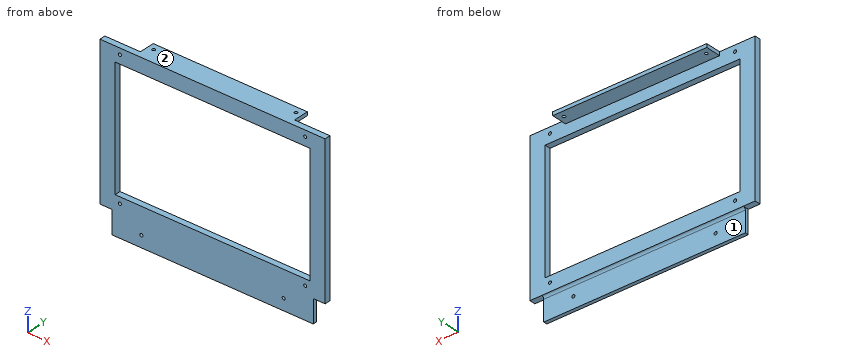
from build123d import *

# Parameters (mm, degrees)
SKETCH1_W           = 170
SKETCH1_H           = 146
BOSS_EXTRUDE1_DEPTH = 3
SKETCH2_R           = 1.3
CUT_EXTRUDE1_DEPTH  = 3
CUT_EXTRUDE2_DEPTH  = 3
BOSS_EXTRUDE2_START = 2
SKETCH4_R           = 1.3
SKETCH4_W           = 164.3
SKETCH4_H           = 101.7
BOSS_EXTRUDE2_DEPTH = 2
BOSS_EXTRUDE5_DEPTH = 10
SKETCH10_W          = 126.5
SKETCH10_H          = 5
BOSS_EXTRUDE6_DEPTH = 10
SKETCH12_W          = 190
SKETCH12_H          = 3
BOSS_EXTRUDE8_DEPTH = 13
SKETCH13_R          = 1.3
CUT_EXTRUDE3_DEPTH  = 13
FILLET4_R           = 2
SKETCH14_R          = 1.3
CUT_EXTRUDE4_DEPTH  = 13
SKETCH15_W          = 30
SKETCH15_H          = 3
CUT_EXTRUDE5_DEPTH  = 13


with BuildPart() as part:
    # Sketch1 → Boss-Extrude1 (new body)
    with BuildSketch(Plane(origin=(0, 0, 0), x_dir=(1, 0, 0), z_dir=(0, 1, 0))):
        Rectangle(SKETCH1_W, SKETCH1_H)
    extrude(amount=BOSS_EXTRUDE1_DEPTH)

    # Sketch2 → Cut-Extrude1 (cut)
    with BuildSketch(Plane(origin=(0, 3, 0), x_dir=(1, 0, 0), z_dir=(0, 1, 0))):
        with Locations(Location((78.15, -67.9, 0), (0, 0, 270))):
            Circle(SKETCH2_R)
        with Locations(Location((-78.15, 46.4, 0), (0, 0, 270))):
            Circle(SKETCH2_R)
        with Locations(Location((-78.15, -67.9, 0), (0, 0, 270))):
            Circle(SKETCH2_R)
        with Locations(Location((78.15, 46.4, 0), (0, 0, 270))):
            Circle(SKETCH2_R)
    extrude(amount=-CUT_EXTRUDE1_DEPTH, mode=Mode.SUBTRACT)

    # Sketch3 → Cut-Extrude2 (cut)
    with BuildSketch(Plane(origin=(0, 3, 0), x_dir=(1, 0, 0), z_dir=(0, 1, 0))):
        Polygon((-78.15, -60.6), (-82.15, -60.6), (-82.15, 41.1), (-78.15, 41.1), (78.15, 41.1), (82.15, 41.1), (82.15, -60.6), (78.15, -60.6), align=None)
    extrude(amount=-CUT_EXTRUDE2_DEPTH, mode=Mode.SUBTRACT)

    # Sketch4 → Boss-Extrude2 (add)
    with BuildSketch(Plane(origin=(0, 3, 0), x_dir=(1, 0, 0), z_dir=(0, 1, 0)).offset(BOSS_EXTRUDE2_START)):
        Polygon((-82.15, 53.5), (85, 53.5), (85, -73), (-85, -73), (-85, 53.5), align=None)
        with Locations(Location((-78.15, 46.4, 0), (0, 0, 270))):
            Circle(SKETCH4_R, mode=Mode.SUBTRACT)
        with Locations(Location((-78.15, -67.9, 0), (0, 0, 270))):
            Circle(SKETCH4_R, mode=Mode.SUBTRACT)
        with Locations(Location((78.15, -67.9, 0), (0, 0, 270))):
            Circle(SKETCH4_R, mode=Mode.SUBTRACT)
        with Locations(Location((78.15, 46.4, 0), (0, 0, 270))):
            Circle(SKETCH4_R, mode=Mode.SUBTRACT)
        with Locations((0, -9.75)):
            Rectangle(SKETCH4_W, SKETCH4_H, mode=Mode.SUBTRACT)
    extrude(amount=-BOSS_EXTRUDE2_DEPTH)

    # Sketch9 → Boss-Extrude5 (add)
    with BuildSketch(Plane.ZY.offset(85)):
        Polygon((-53.5, 3), (-53.5, 5), (73, 5), (73, 0), (-53.5, 0), align=None)
    extrude(amount=BOSS_EXTRUDE5_DEPTH)

    # Sketch10 → Boss-Extrude6 (add)
    with BuildSketch(Plane(origin=(85, 0, 0), x_dir=(0, 0, -1), z_dir=(1, 0, 0))):
        with Locations((-9.75, 2.5)):
            Rectangle(SKETCH10_W, SKETCH10_H)
    extrude(amount=BOSS_EXTRUDE6_DEPTH)

    # Sketch12 → Boss-Extrude8 (add)
    with BuildSketch(Plane(origin=(0, 5, 0), x_dir=(1, 0, 0), z_dir=(0, 1, 0))):
        with Locations((0, -71.5)):
            Rectangle(SKETCH12_W, SKETCH12_H)
    extrude(amount=BOSS_EXTRUDE8_DEPTH)

    # Sketch13 → Cut-Extrude3 (cut)
    with BuildSketch(Plane(origin=(0, 3, 0), x_dir=(1, 0, 0), z_dir=(0, 1, 0))):
        with Locations(Location((-60, 63.25, 0), (0, 0, 270))):
            Circle(SKETCH13_R)
        with Locations(Location((60, 63.25, 0), (0, 0, 270))):
            Circle(SKETCH13_R)
    extrude(amount=-CUT_EXTRUDE3_DEPTH, mode=Mode.SUBTRACT)

    # Fillet4
    fillet4_edges = [part.edges().sort_by_distance(p)[0] for p in [
        (0, 3, -53.5),
    ]]
    fillet(fillet4_edges, radius=FILLET4_R - 0.0001)  # a hair under: the kernel refuses the full size

    # Sketch14 → Cut-Extrude4 (cut)
    with BuildSketch(Plane(origin=(0, 0, 70), x_dir=(-1, 0, 0), z_dir=(0, 0, -1))):
        with Locations((-60, 12.5)):
            Circle(SKETCH14_R)
        with Locations((60, 12.5)):
            Circle(SKETCH14_R)
    extrude(amount=-CUT_EXTRUDE4_DEPTH, mode=Mode.SUBTRACT)

    # Sketch15 → Cut-Extrude5 (cut)
    with BuildSketch(Plane(origin=(0, 18, 0), x_dir=(1, 0, 0), z_dir=(0, 1, 0))):
        with Locations((80, -71.5)):
            Rectangle(SKETCH15_W, SKETCH15_H)
        with Locations((-80, -71.5)):
            Rectangle(SKETCH15_W, SKETCH15_H)
    extrude(amount=-CUT_EXTRUDE5_DEPTH, mode=Mode.SUBTRACT)


solid = part.part
CAD build for the part. Positions are in the model's coordinates, mm. Face numbers are marked on the shaded views. A direction names the side the tool comes from. Give positions to 0.01 mm unless a question says otherwise; leave off trailing zeros. Order: outer loops, then holes, each group sorted by start corner. A loop starts at its lowest first (then second) coordinate and runs counter-clockwise, first axis right, second up. Notation, with made-up numbers: (83.25, -17.75) - (109.25, -17.75) arc R22 cw to (109.25, 12.25) - close; hole circle Ø8 at (20.5, -17.75). An arc over 180 degrees is marked (long way). Write each question's results on one line, items separated by ' | '.
1. Pin check, flat tips, straight feed: pin 1 (3.5 mm diameter, centred on y = 10, z = 71, fed in from -X); pin 2 (1.5 mm diameter, centred on x = 57.5, y = 14, fed in from -Z); pin 3 (1.5 mm diameter, centred on x = 35, y = 5.5, fed in from -Z). Stop position of each tip, or through.
Calculated:
pin 1: stops at x = -65 | pin 2: stops at z = 70 | pin 3: stops at z = -53.52
2. 3-axis set-ups, long thin cutter, end or side, ignore diameter. For the marked faces 1 and 2: which of +Z, -Z, +X, -X, +Y, -Y reach the whole face in a straight line?
Calculated:
face 1: -Z, +X, -X, +Y | face 2: +Z, +X, -X, +Y, -Y
3. Saw through at D-D on z = -58. List the corners of the cut face in (x, y).
Calculated:
outline: (-85, 0) - (85, 0) - (85, 3) - (-85, 3) - close
4. Probe L1, parallel to X at y = 1.35, z = 67.9; L2, parallel to Z at x = 78.15, y = 1.7; L3, parallel to X at y = 2, z = -23. List the from-to ranges inside material, lowest first. Write a range as from..to.
Calculated:
L1: x = -95..-79.45, -76.85..76.85, 79.45..95 | L2: z = -73..-47.7, -45.1..-41.1, 60.6..66.6, 69.2..73 | L3: x = -95..-82.15, 82.15..95
5. Saw through at B-B on z = 27.5. List the corners of the cut face in (x, y).
Calculated:
outline: (-95, 0) - (-82.15, 0) - (-82.15, 5) - (-95, 5) - close; (82.15, 0) - (95, 0) - (95, 5) - (82.15, 5) - close
